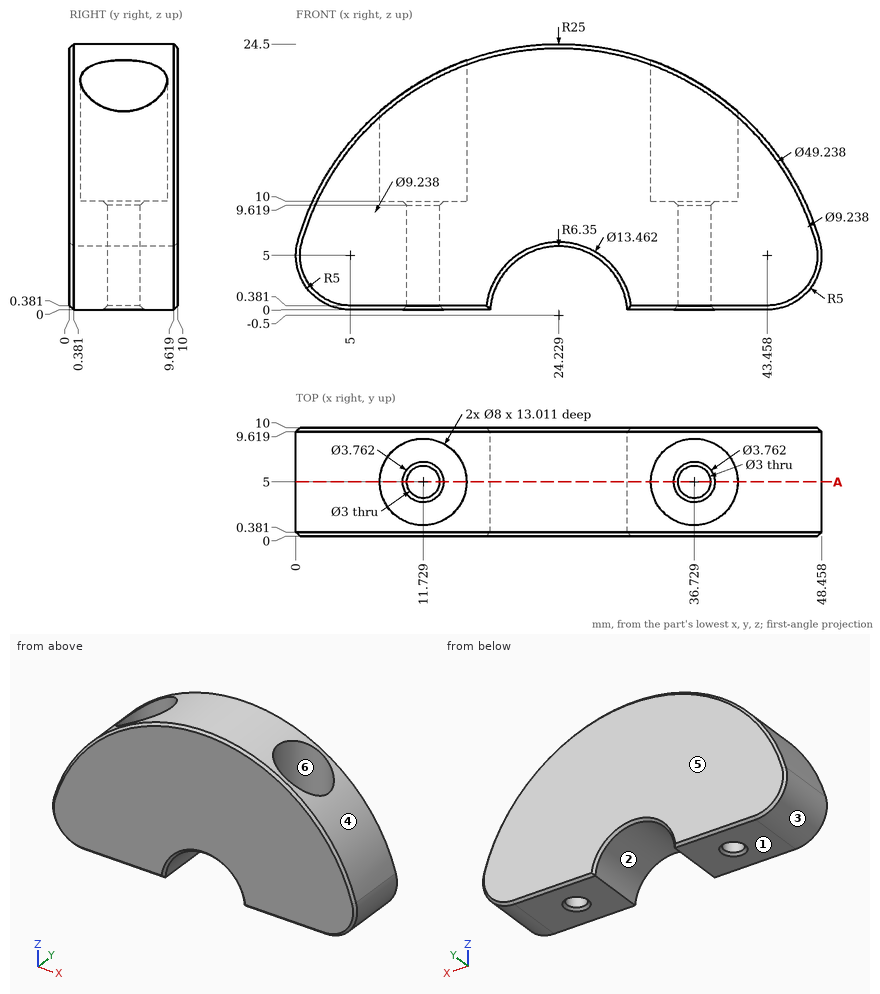
Source: three-view drawing plus pictorial views. Frame: mm from the lowest corner of the part. A direction names the side the tool comes from. Give positions to 0.01 mm unless a question says otherwise; leave off trailing zeros.
1. Section A-A on y = 5. Give the number of separate pieces and of enclosed holes in the cut face, and give its area (3 significant figures).
Derived:
separate pieces: 3
enclosed holes: 0
area: 647 mm2
2. Pin query (flat end, axial travel): pin 1 (3.5 mm diameter, centred on x = 11.73, y = 5, fed in from +Z); pin 2 (1 mm diameter, centred on y = 6.5, z = 16.5, fed in from -X); pin 3 (3 mm diameter, centred on x = 21, y = 4.5, fed in from +Z). Return the tip coordinate at first contact, or that it passes through.
Derived:
pin 1: stops at z = 9.87
pin 2: stops at x = 5.45
pin 3: stops at z = 24.44
3. Mould query, pull axis X, two halves, no side actions, for the marked faces 1, 2, 3 and 4. Classes: released by +X, released by -X, zero draft, split by the parting line, or undercut.
Derived:
face 1: zero draft
face 2: undercut
face 3: released by -X
face 4: split by the parting line
4. Material intervals for L1, parallel to X at y = 6.25, z = 14.5; L2, parallel to X at y = 4.5, z = 16.5; L3, parallel to Z at x = 10, y = 8.25, sorted ascending.
Derived:
L1: x = 4.23 to 7.93, 15.53 to 32.93, 40.53 to 44.23
L2: x = 5.9 to 7.76, 15.7 to 32.76, 40.7 to 42.56
L3: z = 0 to 10
5. Reachability of the marked faces 5 and 6 from +Z, -Z, +X, -X, +Y, -Y: full face, straight path, thin tool, end or side. Return the list, or none.
Derived:
face 5: +Z, -Z, +X, -X, +Y
face 6: +Z
